Could you check a few things on this model? Use its own coordinates, in mm. Give positions to 0.01 mm unless a question says otherwise; leave off trailing zeros. Write each loop counter-clockwise with the first axis right and the second up, starting at its lowest first coordinate (ties: lowest second). Pieces come first, ordered by that corner, then holes. Notation, with made-up numbers: M 30.5,-38.5 L 62.5,-38.5 A26 cw 62.5,-4.5 Z; hole C 48.5,0 d10. An arc over 180 degrees is marked long. One line per item, written item: value.
```python
from build123d import *

# Parameters (mm, degrees)
ESQUISSE1_W             = 90
ESQUISSE1_H             = 2
BASE_EXTRUSION_DEPTH    = 264
ESQUISSE2_W             = 33
ESQUISSE2_H             = 29
ENL_V_MAT_EXTRU_1_DEPTH = 279.92651362
ENL_V_MAT_EXTRU_2_DEPTH = 279.92651362
ESQUISSE4_R             = 1.6
ESQUISSE4_R_2           = 1.7
ESQUISSE4_R_3           = 1.25
ENL_V_MAT_EXTRU_3_DEPTH = 279.92651362
CONG_1_R                = 5
CHANFREIN1_SIZE         = 0.2


with BuildPart() as part:
    # Esquisse1 → Base-Extrusion (new body)
    with BuildSketch(Plane.XY):
        with Locations((45, 1)):
            Rectangle(ESQUISSE1_W, ESQUISSE1_H)
    extrude(amount=BASE_EXTRUSION_DEPTH)

    # Esquisse2 → Enlèv. mat.-Extru.1 (cut, through all)
    with BuildSketch(Plane(origin=(0, 2, 0), x_dir=(-1, 0, 0), z_dir=(0, 1, 0))):
        with Locations((-65, 218)):
            Rectangle(ESQUISSE2_W, ESQUISSE2_H)
    extrude(amount=-ENL_V_MAT_EXTRU_1_DEPTH, mode=Mode.SUBTRACT)

    # Esquisse3 → Enlèv. mat.-Extru.2 (cut, through all)
    with BuildSketch(Plane(origin=(0, 2, 0), x_dir=(-1, 0, 0), z_dir=(0, 1, 0))):
        with BuildLine():
            Line((-27.1, 98.770616019), (-27.1, 62.229383981))
            ThreePointArc((-27.1, 62.229383981), (-26.206969024, 60.314272874), (-24.165879556, 59.767364599))
            Line((-24.165879556, 59.767364599), (-17.765879556, 60.895857275))
            ThreePointArc((-17.765879556, 60.895857275), (-16.284888892, 61.750907634), (-15.7, 63.357876658))
            Line((-15.7, 63.357876658), (-15.7, 97.642123342))
            ThreePointArc((-15.7, 97.642123342), (-16.284888892, 99.249092366), (-17.765879556, 100.104142725))
            Line((-17.765879556, 100.104142725), (-24.165879556, 101.232635401))
            ThreePointArc((-24.165879556, 101.232635401), (-26.206969024, 100.685727126), (-27.1, 98.770616019))
        make_face()
    extrude(amount=-ENL_V_MAT_EXTRU_2_DEPTH, mode=Mode.SUBTRACT)

    # Esquisse4 → Enlèv. mat.-Extru.3 (cut, through all)
    with BuildSketch(Plane(origin=(0, 2, 0), x_dir=(-1, 0, 0), z_dir=(0, 1, 0))):
        with Locations(Location((-22.4, 104.02, 0), (0, 0, 270))):
            Circle(ESQUISSE4_R)
        with Locations(Location((-22.4, 56.98, 0), (0, 0, 270))):
            Circle(ESQUISSE4_R)
        with Locations(Location((-85, 252.5, 0), (0, 0, 270))):
            Circle(ESQUISSE4_R_2)
        with Locations(Location((-85, 11.5, 0), (0, 0, 270))):
            Circle(ESQUISSE4_R_2)
        with Locations(Location((-7.82, 12.49, 0), (0, 0, 270))):
            Circle(ESQUISSE4_R_2)
        with Locations(Location((-7.82, 251.51, 0), (0, 0, 270))):
            Circle(ESQUISSE4_R_2)
        with Locations(Location((-65, 236, 0), (0, 0, 270))):
            Circle(ESQUISSE4_R_3)
        with Locations(Location((-65, 200, 0), (0, 0, 270))):
            Circle(ESQUISSE4_R_3)
    extrude(amount=-ENL_V_MAT_EXTRU_3_DEPTH, mode=Mode.SUBTRACT)

    # Congé1
    cong_1_edges = [part.edges().sort_by_distance(p)[0] for p in [
        (0, 1, 0),
        (0, 1, 264),
        (90, 1, 0),
        (90, 1, 264),
    ]]
    fillet(cong_1_edges, radius=CONG_1_R)

    # Chanfrein1
    chanfrein1_edges = [part.edges().sort_by_distance(p)[0] for p in [
        (0, 0, 132),
        (1.464466094, 0, 1.464466094),
        (1.464466094, 0, 262.535533906),
        (45, 0, 0),
        (45, 0, 264),
        (88.535533906, 0, 1.464466094),
        (88.535533906, 0, 262.535533906),
        (90, 0, 132),
        (7.82, 0, 253.21),
        (65, 0, 237.25),
        (81.5, 0, 218),
        (65, 0, 203.5),
        (65, 0, 232.5),
        (48.5, 0, 218),
        (65, 0, 201.25),
        (85, 0, 254.2),
        (22.4, 0, 105.62),
        (27.1, 0, 80.5),
        (26.206969024, 0, 100.685727126),
        (26.206969024, 0, 60.314272874),
        (20.965879556, 0, 100.668389063),
        (20.965879556, 0, 60.331610937),
        (16.284888892, 0, 99.249092366),
        (16.284888892, 0, 61.750907634),
        (15.7, 0, 80.5),
        (22.4, 0, 58.58),
        (7.82, 0, 14.19),
        (85, 0, 13.2),
        (0, 2, 132),
        (1.464466094, 2, 1.464466094),
        (1.464466094, 2, 262.535533906),
        (45, 2, 0),
        (45, 2, 264),
        (88.535533906, 2, 1.464466094),
        (88.535533906, 2, 262.535533906),
        (90, 2, 132),
        (7.82, 2, 253.21),
        (65, 2, 237.25),
        (81.5, 2, 218),
        (65, 2, 203.5),
        (65, 2, 232.5),
        (48.5, 2, 218),
        (65, 2, 201.25),
        (85, 2, 254.2),
        (22.4, 2, 105.62),
        (27.1, 2, 80.5),
        (26.206969024, 2, 100.685727126),
        (26.206969024, 2, 60.314272874),
        (20.965879556, 2, 100.668389063),
        (20.965879556, 2, 60.331610937),
        (16.284888892, 2, 99.249092366),
        (16.284888892, 2, 61.750907634),
        (15.7, 2, 80.5),
        (22.4, 2, 58.58),
        (7.82, 2, 14.19),
        (85, 2, 13.2),
    ]]
    chamfer(chanfrein1_edges, length=CHANFREIN1_SIZE)


solid = part.part
```
1) I'm going to push flat-ended pins straight in: pin 1 (2.5 mm diameter, centred on x = 85, z = 11.5, fed in from -Y) (3 decimals); pin 2 (3.5 mm diameter, centred on x = 22.4, z = 104.02, fed in from +Y). Where does each tip first touch, or does it pass through?
Outcome:
pin 1: passes through
pin 2: stops at y = 1.95
2) Please list where these lines run through material, in increasing order: L1, parallel to Z at x = 85, y = 0.85; L2, parallel to Z at x = 18, y = 0.3; L3, parallel to X at y = 0.4, z = 229. Write a range as from..to.
Outcome:
L1: z = 0..9.8, 13.2..250.8, 254.2..264
L2: z = 0..60.85, 100.15..264
L3: x = 0..48.5, 81.5..90
3) If we section it at A-A, the plane z = 71: Write out the boundary of the cut face in (x, y).
Outcome:
outline: M 0,0.2 L 0.2,0 L 15.5,0 L 15.7,0.2 L 15.7,1.8 L 15.5,2 L 0.2,2 L 0,1.8 Z; M 27.1,0.2 L 27.3,0 L 89.8,0 L 90,0.2 L 90,1.8 L 89.8,2 L 27.3,2 L 27.1,1.8 Z
4) If we section it at B-B, the plane y = 0.9: Give the number of separate pieces and of enclosed holes in the cut face, then the cut area to 3 significant figures.
Outcome:
separate pieces: 1
enclosed holes: 10
area: 22,300 mm^2
